from build123d import *

# Parameters (mm, degrees)
BOSS_EXTRUDE1_DEPTH = 25.4
SKETCH2_W           = 3.175
SKETCH2_H           = 42.291
BOSS_EXTRUDE2_DEPTH = 21.2344
SKETCH3_W           = 12.0396
SKETCH3_H           = 1.5494
BOSS_EXTRUDE3_DEPTH = 13.462
SKETCH4_R           = 2.49555
CUT_EXTRUDE1_DEPTH  = 16.51
SKETCH5_W           = 9.2202
SKETCH5_H           = 10.16
CUT_EXTRUDE2_DEPTH  = 6.35
SKETCH6_W           = 9.2202
SKETCH6_H           = 10.16
CUT_EXTRUDE3_DEPTH  = 6.35


with BuildPart() as part:
    # Sketch1 → Boss-Extrude1 (new body)
    with BuildSketch(Plane.XY):
        Polygon((28.5369, 30.1371), (35.3695, 30.1371), (35.3695, -30.1371), (-35.3695, -30.1371), (-35.3695, -21.4503), (-43.6753, -21.4503), (-43.6753, 20.5867), (-35.3695, 20.5867), (-35.3695, 30.1371), (-28.0035, 30.1371), (-28.0035, 34.8869), (6.6167, 34.8869), (6.6167, 45.0469), (15.8369, 45.0469), (15.8369, 34.8869), (28.5369, 34.8869), align=None)
    extrude(amount=BOSS_EXTRUDE1_DEPTH)

    # Sketch2 → Boss-Extrude2 (add)
    with BuildSketch(Plane(origin=(35.3695, 0, 0), x_dir=(0, 0, -1), z_dir=(1, 0, 0))):
        with Locations((-3.1115, -1.11983587)):
            Rectangle(SKETCH2_W, SKETCH2_H)
    extrude(amount=BOSS_EXTRUDE2_DEPTH)

    # Sketch3 → Boss-Extrude3 (add)
    with BuildSketch(Plane(origin=(35.3695, 0, 0), x_dir=(0, 0, -1), z_dir=(1, 0, 0))):
        with Locations((-14.5796, 1.4478)):
            Rectangle(SKETCH3_W, SKETCH3_H)
    extrude(amount=BOSS_EXTRUDE3_DEPTH)

    # Sketch4 → Cut-Extrude1 (cut)
    with BuildSketch(Plane(origin=(0, 2.2225, 0), x_dir=(1, 0, 0), z_dir=(0, 1, 0))):
        with Locations(Location((43.82135, -14.5796, 0), (0, 0, 270))):
            Circle(SKETCH4_R)
    extrude(amount=-CUT_EXTRUDE1_DEPTH, mode=Mode.SUBTRACT)

    # Sketch5 → Cut-Extrude2 (cut)
    with BuildSketch(Plane.XY.offset(25.4)):
        with Locations((11.2268, 39.9669)):
            Rectangle(SKETCH5_W, SKETCH5_H)
    extrude(amount=-CUT_EXTRUDE2_DEPTH, mode=Mode.SUBTRACT)

    # Sketch6 → Cut-Extrude3 (cut)
    with BuildSketch(Plane(origin=(0, 0, 0), x_dir=(-1, 0, 0), z_dir=(0, 0, -1))):
        with Locations((-11.2268, 39.9669)):
            Rectangle(SKETCH6_W, SKETCH6_H)
    extrude(amount=-CUT_EXTRUDE3_DEPTH, mode=Mode.SUBTRACT)


solid = part.part
Work out the finished part from the listing and answer in its coordinate system (mm). A direction names the side the tool comes from. Round coordinates to 2 decimals unless told otherwise and drop trailing zeros. Loops run counter-clockwise (first coordinate to the right, second up) from the corner with the lowest first, then second, coordinate; pieces in that order, holes last. Notation, with made-up numbers: M -20.75,17.5 L -12.75,17.5 A9 cw -12.75,21.5 Z; hole C 6.5,57 d8. An arc over 180 degrees is marked long. One line per question, with ' | ' between items. Start each with the question number.
(1) A cutting plane is placed at A-A on y = 5.5. Write down the section's boundary in (x, z), plus the area to 3 significant figures.
(2) For a pull along X with two mould halves and no side action, classify faces 1 (the face through (28.537, 33, 13)), 2 (the face through (46, -22.265, 3)), 3 (the face through (41.385, 1.459, 14.039)) as released by +X, released by -X, zero draft, split by the parting line, or undercut.
(3) A cutting plane is placed at B-B on z = 21.75. Write down the section's boundary in (x, y), plus the area to 3 significant figures.
(4) A cutting plane is placed at C-C on x = 12. Write down the section's boundary in (y, z).
(5) A cutting plane is placed at D-D on x = 32. Write down the section's boundary in (y, z), plus the area to 3 significant figures.
(6) Flat-ended cylindrical pins translate along their axes: pin 1 Ø4 at (x, z) = (39, 7) entering from +Y; pin 2 Ø23.5 at (x, y) = (50, 4.5) entering from -Z; pin 3 Ø0.8 at (x, y) = (40.5, 1.5) entering from +Z. Find the tip coordinate at first contact, or state that the pin passes through.
(7) Find the intervals of material crossed by line 1 (Y direction, x = 23.5, z = 19.25); line 2 (X direction, y = -1, z = 16.25); line 3 (Y direction, x = -32, z = 10), in increasing order.
(8) A tool of negligible diameter and unlimited length cuts with its end or side. For faces 4 (the face through (11, 40, 6.35)), 5 (the face through (-40, 20.587, 13)), 6 (the face through (11, 40, 19.05)), from which of +Z, -Z, +X, -X, +Y, -Y can it reach the whole face along a straight path? Write none if from no direction.
Geometry check:
1) outline: M -43.68,0 L 35.37,0 L 35.37,1.52 L 56.6,1.52 L 56.6,4.7 L 35.37,4.7 L 35.37,25.4 L -43.68,25.4 Z | area: 2,080 mm²
2) face 1: released by +X | face 2: zero draft | face 3: undercut
3) outline: M -43.68,-21.45 L -35.37,-21.45 L -35.37,-30.14 L 35.37,-30.14 L 35.37,30.14 L 28.54,30.14 L 28.54,34.89 L -28,34.89 L -28,30.14 L -35.37,30.14 L -35.37,20.59 L -43.68,20.59 Z | area: 4,880 mm²
4) outline: M -30.14,0 L 34.89,0 L 34.89,6.35 L 45.05,6.35 L 45.05,19.05 L 34.89,19.05 L 34.89,25.4 L -30.14,25.4 Z
5) outline: M -30.14,0 L 30.14,0 L 30.14,25.4 L -30.14,25.4 Z | area: 1,530 mm²
6) pin 1: stops at y = 2.22 | pin 2: stops at z = 1.52 | pin 3: stops at z = 20.6
7) line 1: y = -30.14 to 34.89 | line 2: x = -43.68 to 35.37 | line 3: y = -30.14 to 30.14
8) face 4: -Z, +X, -X, +Y | face 5: +Z, -Z, -X, +Y | face 6: +Z, +X, -X, +Y
